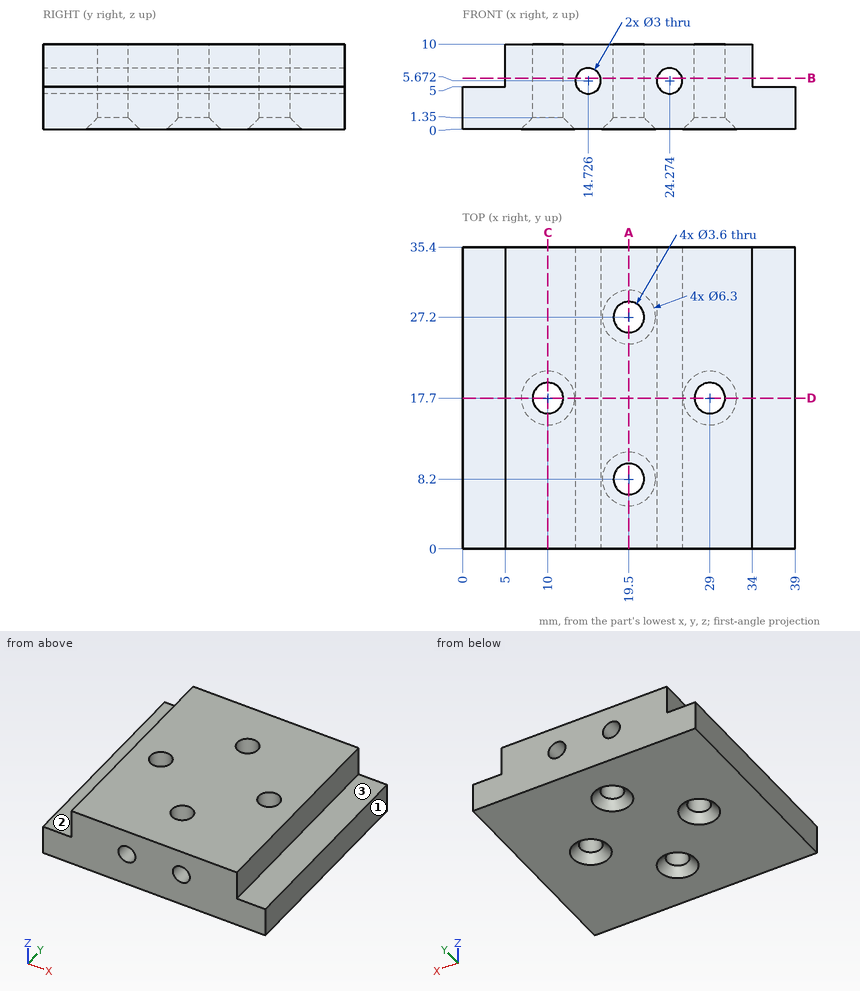
Job drawing, mm, ordinate dimensions from the low corner. One solid piece. A direction names the side the tool comes from. Give positions to 0.01 mm unless a question says otherwise; leave off trailing zeros. Order: outer loops, then holes, each group sorted by start corner. A loop starts at its lowest first (then second) coordinate and runs counter-clockwise, first axis right, second up. Notation, with made-up numbers: M -21.5,37 L 30.5,37 A31 cw 30.5,75 Z; hole C -24,-14.75 d3. An arc over 180 degrees is marked long. Return JSON: item names as keys, results as strings.
Q1. Band-saw the part on B-B (z = 6). Give the cut face in (x, y).
Answer list:
{"outline": "M 5,0 L 13.26,0 L 13.26,35.4 L 5,35.4 Z; M 16.19,0 L 22.81,0 L 22.81,35.4 L 16.19,35.4 Z; M 25.74,0 L 34,0 L 34,35.4 L 25.74,35.4 Z; hole C 10,17.7 d3.6; hole C 19.5,8.2 d3.6; hole C 19.5,27.2 d3.6; hole C 29,17.7 d3.6"}
Q2. Band-saw the part on D-D (y = 17.7). Give the cut face in (x, z), then the cut area to 3 significant figures.
Answer list:
{"outline": "M 0,0 L 6.85,0 L 8.2,1.35 L 8.2,10 L 5,10 L 5,5 L 0,5 Z; M 11.8,1.35 L 13.15,0 L 25.85,0 L 27.2,1.35 L 27.2,10 L 11.8,10 Z; M 30.8,1.35 L 32.15,0 L 39,0 L 39,5 L 34,5 L 34,10 L 30.8,10 Z; hole C 14.73,5.67 d3; hole C 24.27,5.67 d3", "area": "250 mm^2"}
Q3. Flat gauge pins, fed straight in: pin 1 (4.5 mm diameter, centred on x = 29, y = 17.7, fed in from -Z); pin 2 (5 mm diameter, centred on y = 18.5, z = 9, fed in from +X); pin 3 (1 mm diameter, centred on y = 14.5, z = 9, fed in from -X). Where does each tip first touch, or does it go through?
Answer list:
{"pin 1": "stops at z = 0.9", "pin 2": "stops at x = 34", "pin 3": "stops at x = 5"}
Q4. 3-axis set-ups, long thin cutter, end or side, ignore diameter. For the marked faces 1, 2 and 3: which of +Z, -Z, +X, -X, +Y, -Y reach the whole face in a straight line?
Answer list:
{"face 1": "+Z, -Z, +X, +Y, -Y", "face 2": "+Z, -X, +Y, -Y", "face 3": "+Z, +X, +Y, -Y"}
Q5. Band-saw the part on A-A (x = 19.5). Give the cut face in (y, z).
Answer list:
{"outline": "M 0,0 L 5.05,0 L 6.4,1.35 L 6.4,10 L 0,10 Z; M 10,1.35 L 11.35,0 L 24.05,0 L 25.4,1.35 L 25.4,10 L 10,10 Z; M 29,1.35 L 30.35,0 L 35.4,0 L 35.4,10 L 29,10 Z"}
Q6. Wall check: probe 1 along Y at (x, z) = (10, 4.5); probe 2 along Y at (x, z) = (19.5, 3.25); probe 3 along X at (y, z) = (13, 6.25). Give the ranges that are in metal, low to high. Write a range as from..to.
Answer list:
{"probe 1": "y = 0..15.9, 19.5..35.4", "probe 2": "y = 0..6.4, 10..25.4, 29..35.4", "probe 3": "x = 5..13.34, 16.11..22.89, 25.66..34"}
Q7. Band-saw the part on C-C (x = 10). Give the cut face in (y, z).
Answer list:
{"outline": "M 0,0 L 14.55,0 L 15.9,1.35 L 15.9,10 L 0,10 Z; M 19.5,1.35 L 20.85,0 L 35.4,0 L 35.4,10 L 19.5,10 Z"}
